Answer from the drawing. Dimensions are ordinates in mm from the lowest x, y and z of the part. Give positions to 0.01 mm unless a question says otherwise; leave off trailing zeros.
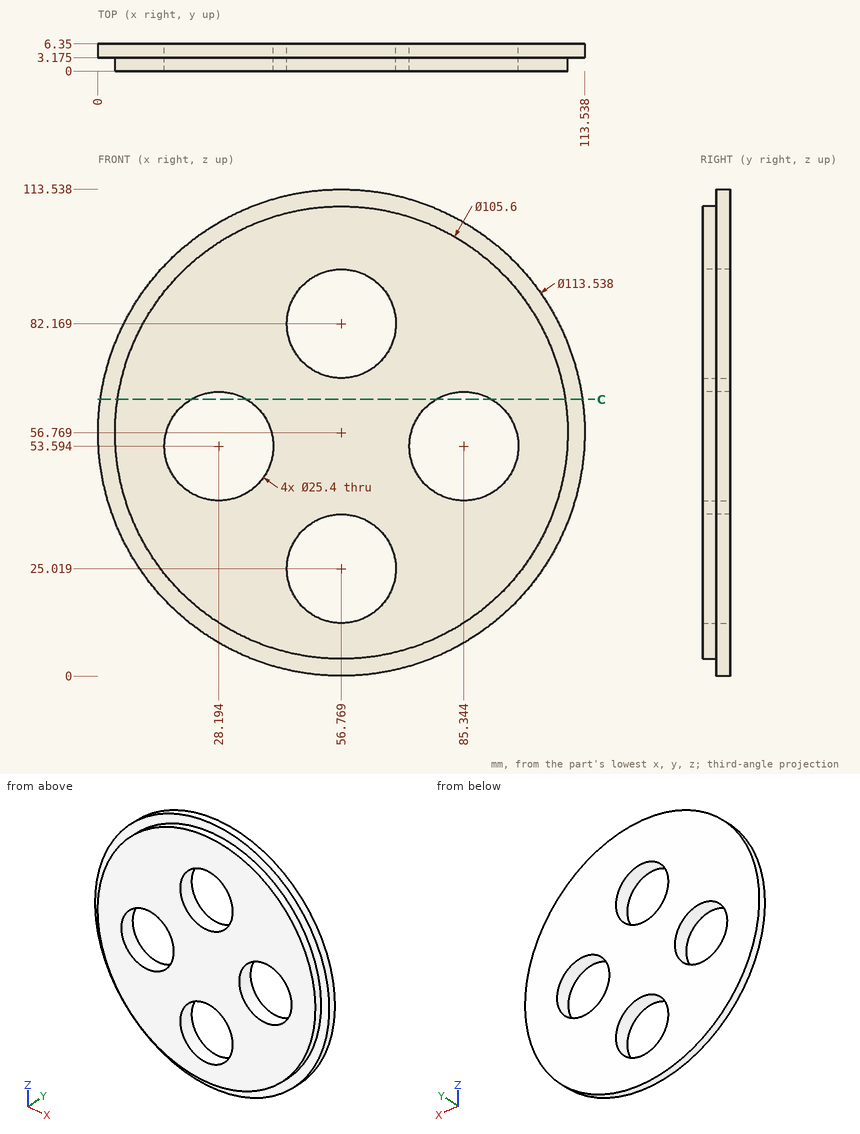
Item 1: Find the intervals of material crossed by line 1 along X through (y, z) = (6, 53.5) (1 decimal); line 2 along X through (y, z) = (3, 46.5) (1 decimal); line 3 along Z through (x, y) = (28, 3) (1 decimal), in increasing order.
Result set:
line 1: x = 0.1 to 15.5, 40.9 to 72.6, 98 to 113.4
line 2: x = 5 to 17.7, 38.7 to 74.8, 95.9 to 108.6
line 3: z = 12.5 to 40.9, 66.3 to 101
Item 2: Section C-C (z = 64.5) is taken. Give the number of separate pieces and of enclosed holes in the cut face.
Result set:
separate pieces: 3
enclosed holes: 0
Item 3: Each of these flat-tipped pins is pushed along its axis until it touches: pin 1 Ø3 at (x, y) = (29.5, 5.5) entering from +Z; pin 2 Ø10 at (x, z) = (99, 14) entering from -Y (1 decimal); pin 3 Ø3 at (y, z) = (1.5, 21) entering from -X. Where does it stop, or does it pass through?
Result set:
pin 1: stops at z = 107.35
pin 2: stops at y = 3.2
pin 3: stops at x = 16.6
